```python
from build123d import *

# Parameters (mm, degrees)
SKETCH025_R     = 106.066017
SKETCH025_R_2   = 2
SKETCH025_R_3   = 69
PAD011_DEPTH    = 9.5
SKETCH026_R     = 100
SKETCH026_R_2   = 82
POCKET004_DEPTH = 7.5
CHAMFER012_SIZE = 9
CHAMFER013_SIZE = 4


with BuildPart() as part:
    # Sketch025 → Pad011 (new body)
    with BuildSketch(Plane.XY):
        Circle(SKETCH025_R)
        with Locations((-62.25, 62.25)):
            Circle(SKETCH025_R_2, mode=Mode.SUBTRACT)
        with Locations((62.25, 62.25)):
            Circle(SKETCH025_R_2, mode=Mode.SUBTRACT)
        with Locations((62.25, -62.25)):
            Circle(SKETCH025_R_2, mode=Mode.SUBTRACT)
        with Locations((-62.25, -62.25)):
            Circle(SKETCH025_R_2, mode=Mode.SUBTRACT)
        Circle(SKETCH025_R_3, mode=Mode.SUBTRACT)
    extrude(amount=PAD011_DEPTH)

    # Sketch026 → Pocket004 (cut)
    with BuildSketch(Plane.XY):
        Circle(SKETCH026_R)
        Circle(SKETCH026_R_2, mode=Mode.SUBTRACT)
    extrude(amount=POCKET004_DEPTH, mode=Mode.SUBTRACT)

    # Chamfer012
    chamfer012_edges = [part.edges().sort_by_distance(p)[0] for p in [
        (-69, 0, 0),
    ]]
    chamfer(chamfer012_edges, length=CHAMFER012_SIZE)

    # Chamfer013
    chamfer013_edges = [part.edges().sort_by_distance(p)[0] for p in [
        (-106.066017, 0, 0),
    ]]
    chamfer(chamfer013_edges, length=CHAMFER013_SIZE)


with BuildPart() as part_1:
    # Body009 placement: moved
    add(part.part.moved(Location((0, 0, 35))))


solid = part_1.part
```
For this review, take the finished solid that the model builds, in its own axes (mm). A direction names the side the tool comes from. Round coordinates to 2 decimals unless told otherwise and drop trailing zeros. Write each loop counter-clockwise with the first axis right and the second up, starting at its lowest first coordinate (ties: lowest second). Pieces come first, ordered by that corner, then holes. Notation, with made-up numbers: (6, 48) - (17, 48) arc R23 ccw to (17, 63) - close; hole circle Ø7 at (46.25, 12). An arc over 180 degrees is marked (long way). Use CSV: the item, a comma, the result in double quotes.
1) Clearance check with flat-ended pins moving along their axes: pin 1 Ø2.5 at (x, y) = (-62.25, 62.25) entering from -Z; pin 2 Ø5 at (x, y) = (62.25, -62.25) entering from -Z; pin 3 Ø2 at (y, z) = (62.5, 40) entering from -X; pin 4 Ø4 at (y, z) = (-48.5, 39.5) entering from +X. State where each tip first meets the part, or that it passes through.
Conclusion:
pin 1,"passes through"
pin 2,"stops at z = 42.5"
pin 3,"stops at x = -86.42"
pin 4,"stops at x = 95.33"
2) Add section A-A on y = 0. Write out the cut boundary in (x, z), and give its area (3 significant figures).
Conclusion:
outline,"(-106.07, 39) - (-102.07, 35) - (-100, 35) - (-100, 42.5) - (-82, 42.5) - (-82, 35) - (-78, 35) - (-69, 44) - (-69, 44.5) - (-106.07, 44.5) - close; (69, 44) - (78, 35) - (82, 35) - (82, 42.5) - (100, 42.5) - (100, 35) - (102.07, 35) - (106.07, 39) - (106.07, 44.5) - (69, 44.5) - close"
area,"337 mm^2"
3) For faces 1 (the cylindrical face through (-18, -80, 39)), 2 (the flat face through (-1.5, -69.2, 44.5)), list the 3-axis set-ups (+Z, -Z, +X, -X, +Y, -Y) from which the entire face can be reached by the end or side of a thin tool; tool diameter is ignored.
Conclusion:
face 1,"-Z"
face 2,"+Z, +X, -X, +Y, -Y"
4) The part is to be moulded in two halves that separate along Y. For faces 3 (the cylindrical face through (95.38, 30.04, 38.7)), 4 (the conical face through (-22.168, -99.829, 35.194)), 5 (the flat face through (75, -68, 35)), 6 (the flat face through (-8, 82, 42.5)), say which applies: pulls with the +Y half, pulls with the -Y half, needs draft (parallel to the pull), parting line crosses it, or undercut.
Conclusion:
face 3,"undercut"
face 4,"parting line crosses it"
face 5,"needs draft"
face 6,"undercut"
5) Wall thickness on line 1 along Y through (x, z) = (62.25, 44); line 2 along Y through (x, z) = (-39, 36.25); line 3 along X through (y, z) = (-50, 37.5): over which ranges is each line inside the solid? List them lowest first. Write a range as from..to.
Conclusion:
line 1,"y = -85.88..-64.25, -60.25..-29.76, 29.76..60.25, 64.25..85.88"
line 2,"y = -95.67..-92.08, -72.13..-66.1, 66.1..72.13, 92.08..95.67"
line 3,"x = -91.84..-86.6, -64.99..-56.57, 56.57..64.99, 86.6..91.84"
6) Add section C-C on z = 37.25. Write out the cut boundary in (x, y), and give its area (3 significant figures).
Conclusion:
outline,"circle Ø208.63 at (0, 0); circle Ø164 at (0, 0); hole circle Ø200 at (0, 0); hole circle Ø151.5 at (0, 0)"
area,"5,870 mm^2"
